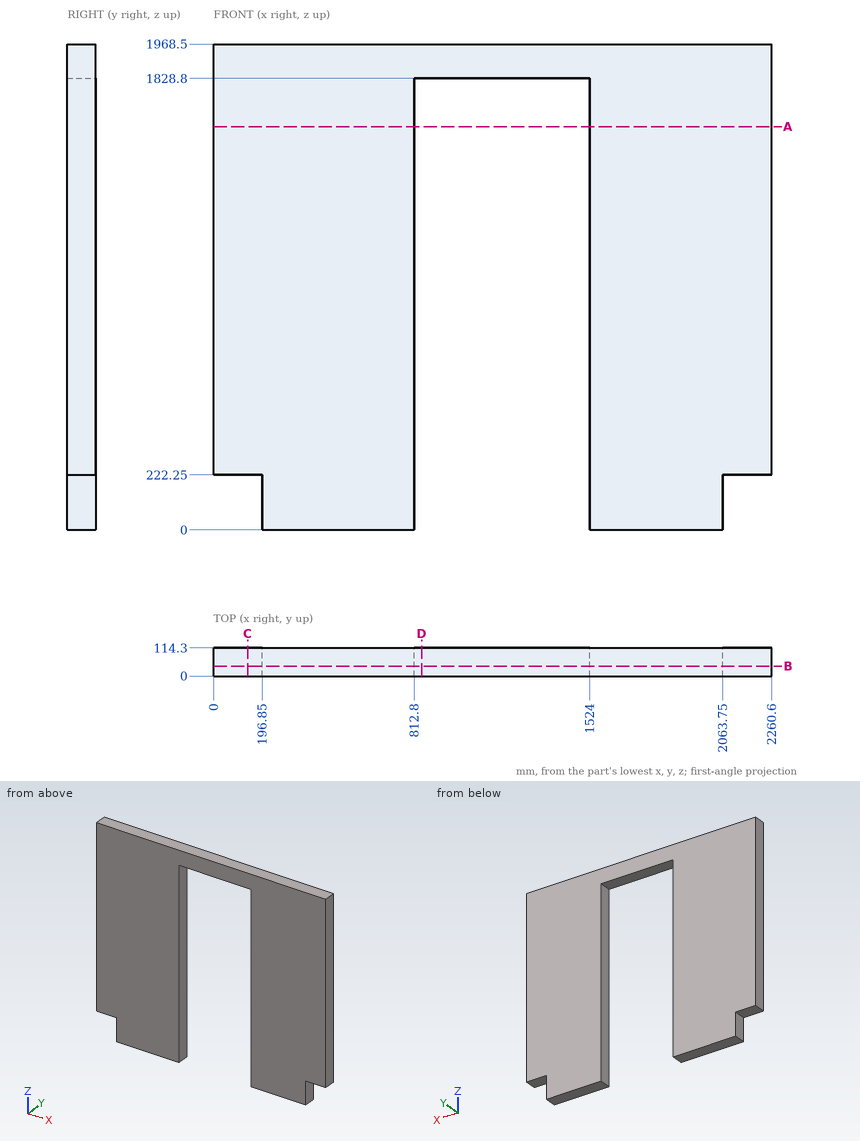
The drawing under review shows one solid part. Ordinate dimensions are in mm from its lowest x, y, z. Coordinates: 2 decimals unless noted, no trailing zeros. Order: outer loops, then holes, each group sorted by start corner. A loop starts at its lowest first (then second) coordinate and runs counter-clockwise, first axis right, second up. Notation, with made-up numbers: M 54,-39 L 86,-39 A17 ccw 86,-10 Z; hole C -33.75,-13 d2. An arc over 180 degrees is marked long. Use a Markdown table: item, result.
(1) Wall thickness on probe 1 along X at (y, z) = (21, 1111); probe 2 along Z at (x, y) = (855, 63.5); probe 3 along Z at (x, y) = (99.5, 100.5): over which ranges is each line inside the solid? List them lowest first.
Worked answers:
| item | result |
|---|---|
| probe 1 | x = 0 to 812.8, 1524 to 2260.6 |
| probe 2 | z = 1828.8 to 1968.5 |
| probe 3 | z = 222.25 to 1968.5 |
(2) For P1, Ø8, axis at x = 1952.5, z = 973, coming from the -Y side, flat-tipped, find the tip position at first contact; note if it passes through.
Worked answers:
| item | result |
|---|---|
| P1 | stops at y = 0 |
(3) Add section D-D (x = 843). Give the boundary of the cut face in (y, z).
Worked answers:
| item | result |
|---|---|
| outline | M 0,1828.8 L 114.3,1828.8 L 114.3,1968.5 L 0,1968.5 Z |
(4) Add section B-B (y = 39.5). Give the boundary of the cut face in (x, z), then the cut area to 3 significant figures.
Worked answers:
| item | result |
|---|---|
| outline | M 0,222.25 L 196.85,222.25 L 196.85,0 L 812.8,0 L 812.8,1828.8 L 1524,1828.8 L 1524,0 L 2063.75,0 L 2063.75,222.25 L 2260.6,222.25 L 2260.6,1968.5 L 0,1968.5 Z |
| area | 3,060,000 mm2 |
(5) Add section C-C (x = 138). Give the boundary of the cut face in (y, z), then the cut area to 3 significant figures.
Worked answers:
| item | result |
|---|---|
| outline | M 0,222.25 L 114.3,222.25 L 114.3,1968.5 L 0,1968.5 Z |
| area | 200,000 mm2 |
(6) Add section A-A (z = 1634). Give the boundary of the cut face in (x, y), then the cut area to 3 significant figures.
Worked answers:
| item | result |
|---|---|
| outline | M 0,0 L 812.8,0 L 812.8,114.3 L 0,114.3 Z; M 1524,0 L 2260.6,0 L 2260.6,114.3 L 1524,114.3 Z |
| area | 177,000 mm2 |
